from build123d import *

# Parameters (mm, degrees)
F0_W     = 1828.8
F0_H     = 38.1
F1_DEPTH = 19.05
F2_W     = 38.1
F2_H     = 38.1
F3_DEPTH = 9.525
F5_DEPTH = 19.051
F6_R     = 3.175


with BuildPart() as f1:
    # F0 (on Front) → F1 (new body)
    with BuildSketch(Plane.XZ):
        Rectangle(F0_W, F0_H)
    extrude(amount=F1_DEPTH)

    # F2 (on face) → F3 (cut)
    with BuildSketch(Plane(origin=(0, 0, 0), x_dir=(-1, 0, 0), z_dir=(0, 1, 0))):
        Rectangle(F2_W, F2_H)
    extrude(amount=-F3_DEPTH, mode=Mode.SUBTRACT)

    # F4 (on face) → F5 (cut, through all)
    with BuildSketch(Plane.XZ.offset(19.05)):
        Polygon((-876.3, -19.05), (-914.4, 19.05), (-914.4, -19.05), align=None)
        Polygon((876.3, -19.05), (914.4, -19.05), (914.4, 19.05), align=None)
    extrude(amount=-F5_DEPTH, mode=Mode.SUBTRACT)

    # F6
    f6_edges = [f1.edges().sort_by_distance(p)[0] for p in [
        (0, -19.05, 19.05),
        (0, -19.05, -19.05),
    ]]
    fillet(f6_edges, radius=F6_R)


solid = f1.part
For this review, take the finished solid that the model builds, in its own axes (mm). Give positions to 0.01 mm unless a question says otherwise; leave off trailing zeros. Loops run counter-clockwise (first coordinate to the right, second up) from the corner with the lowest first, then second, coordinate; pieces in that order, holes last. Notation, with made-up numbers: M 67,69.25 L 118,69.25 A24 cw 118,79.25 Z; hole C 87.25,46.25 d9. An arc over 180 degrees is marked long. Answer as a JSON object with one key per item and string values. Group by question number.
Q1. Insertion check: P1, Ø10, axis at x = 389.5, z = -3.5, coming from the +Y side; P2, Ø3, axis at y = -6.5, z = 2.5, coming from the -X side; P3, Ø10.5, axis at y = -4.5, z = -4, coming from the +X side. Each pin has a flat end and moves straight along its axis. Give the tip position at first contact, or say it passes through.
Q2. Add section B-B on z = 0. Give the boundary of the cut face in (x, y) (3 decimals).
Q3. Mouldability with a two-part tool opening along X and no side actions: class faces 1 (the flat face through (0, -9.525, 0)), 2 (the flat face through (-895.08, -9.66, -0.27)), 3 (the flat face through (895.62, -9.66, 0.27)) as +X half, -X half, draft (parallel to the pull), parting line (faces both ways), or undercut.
Q4. For probe 1 along X at (y, z) = (-7.25, 16); probe 2 along Z at (x, y) = (-831.5, -16.25); probe 3 along Y at (x, z) = (622, 17), list the stretches that pass through material, from the lowest coordinate up. Write a range as [from, to].
Q5. Add section A-A on y = -3. Give the boundary of the cut face in (x, z).
Checked values:
{
 "1": {"P1": "y = 0", "P2": "x = -899.35", "P3": "x = 896.6"},
 "2": {"outline": "M -895.35,-19.05 L 895.35,-19.05 L 895.35,0 L 19.05,0 L 19.05,-9.525 L -19.05,-9.525 L -19.05,0 L -895.35,0 Z"},
 "3": {"face 1": "undercut", "face 2": "-X half", "face 3": "+X half"},
 "4": {"probe 1": "[-911.35, -19.05], [19.05, 911.35]", "probe 2": "[-19.03, 19.03]", "probe 3": "[-18.84, 0]"},
 "5": {"outline": "M -914.4,19.05 L -876.3,-19.05 L -19.05,-19.05 L -19.05,19.05 Z; M 19.05,-19.05 L 876.3,-19.05 L 914.4,19.05 L 19.05,19.05 Z"}
}
